The drawing under review shows one solid part. Ordinate dimensions are in mm from its lowest x, y, z. A direction names the side the tool comes from. Round coordinates to 2 decimals unless told otherwise and drop trailing zeros. Loops run counter-clockwise (first coordinate to the right, second up) from the corner with the lowest first, then second, coordinate; pieces in that order, holes last. Notation, with made-up numbers: M 9.5,-37 L 64.5,-37 A8 ccw 64.5,-23 Z; hole C 50.25,24.5 d11. An arc over 180 degrees is marked long. Use a Markdown table: item, result.
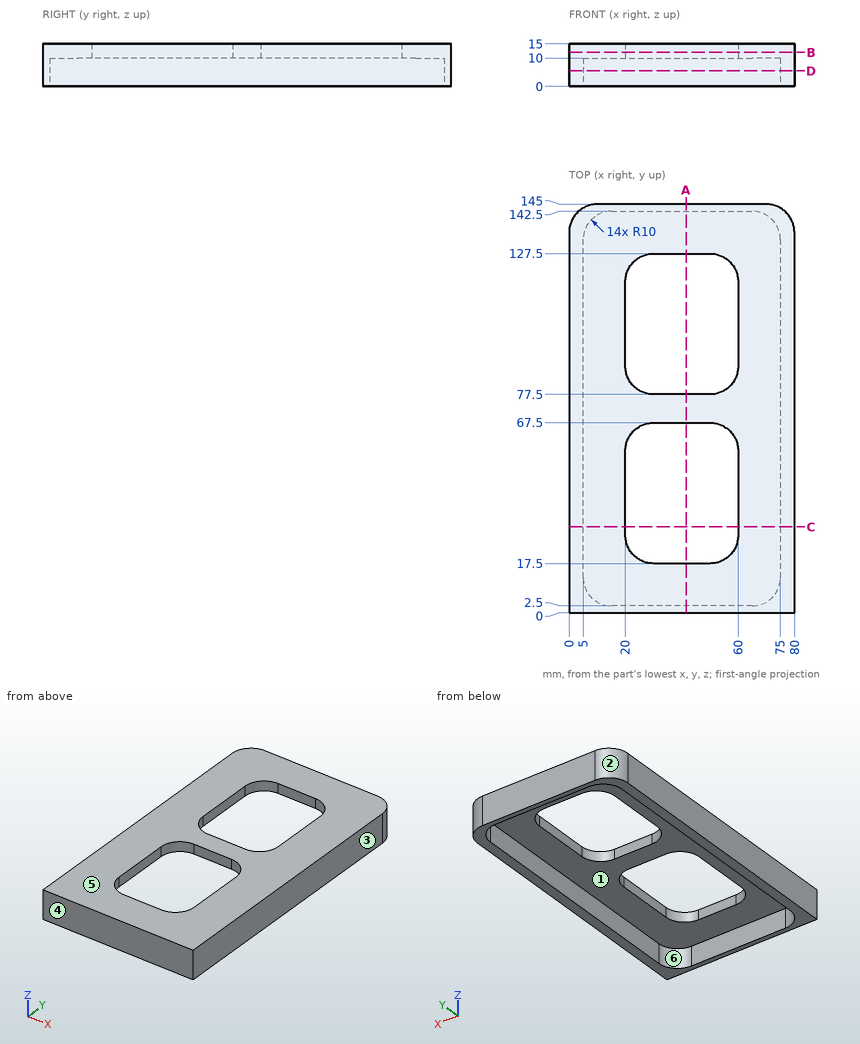
1. Machinability: for the marked faces 5 and 6, which of the approach directions +Z, -Z, +X, -X, +Y, -Y give a long, thin tool a straight path to every point of the face, cutting with its end or side? Answer none if there is none.
Check values:
| item | result |
|---|---|
| face 5 | +Z, +X, -X, +Y, -Y |
| face 6 | -Z |
2. The part is to be moulded in two halves that separate along X. For the marked faces 1, 2, 3 and 4, say which applies: pulls with the +X half, pulls with the -X half, needs draft (parallel to the pull), parting line crosses it, or undercut.
Check values:
| item | result |
|---|---|
| face 1 | undercut |
| face 2 | pulls with the -X half |
| face 3 | pulls with the +X half |
| face 4 | needs draft |
3. Take a section at A-A on x = 41.5. Give the boundary of the cut face in (y, z).
Check values:
| item | result |
|---|---|
| outline | M 0,0 L 2.5,0 L 2.5,10 L 17.5,10 L 17.5,15 L 0,15 Z; M 67.5,10 L 77.5,10 L 77.5,15 L 67.5,15 Z; M 127.5,10 L 142.5,10 L 142.5,0 L 145,0 L 145,15 L 127.5,15 Z |
4. Wall thickness on line 1 along Y through (x, z) = (41, 10.25); line 2 along X through (y, z) = (87.5, 1.5); line 3 along Y through (x, z) = (41, 6.25): over which ranges is each line inside the solid? List them lowest first. Write a range as from..to.
Check values:
| item | result |
|---|---|
| line 1 | y = 0..17.5, 67.5..77.5, 127.5..145 |
| line 2 | x = 0..5, 75..80 |
| line 3 | y = 0..2.5, 142.5..145 |
5. Insertion check: pin 1 (4 mm diameter, centred on x = 22.5, z = 5, fed in from -Y). The pin has a flat end and moves straight along its axis. Give the tip position at first contact, or say it passes through.
Check values:
| item | result |
|---|---|
| pin 1 | stops at y = 0 |
6. Take a section at D-D on z = 5.5. Give the boundary of the cut face in (x, y), and give its area (3 significant figures).
Check values:
| item | result |
|---|---|
| outline | M 0,0 L 80,0 L 80,135 A10 ccw 70,145 L 10,145 A10 ccw 0,135 Z; hole M 5,12.5 A10 ccw 15,2.5 L 65,2.5 A10 ccw 75,12.5 L 75,132.5 A10 ccw 65,142.5 L 15,142.5 A10 ccw 5,132.5 Z |
| area | 1,840 mm² |
7. Take a section at C-C on y = 30.5. Give the boundary of the cut face in (x, z), and give its area (3 significant figures).
Check values:
| item | result |
|---|---|
| outline | M 0,0 L 5,0 L 5,10 L 20,10 L 20,15 L 0,15 Z; M 60,10 L 75,10 L 75,0 L 80,0 L 80,15 L 60,15 Z |
| area | 300 mm² |
8. Take a section at B-B on z = 12. Give the boundary of the cut face in (x, y).
Check values:
| item | result |
|---|---|
| outline | M 0,0 L 80,0 L 80,135 A10 ccw 70,145 L 10,145 A10 ccw 0,135 Z; hole M 20,27.5 A10 ccw 30,17.5 L 50,17.5 A10 ccw 60,27.5 L 60,57.5 A10 ccw 50,67.5 L 30,67.5 A10 ccw 20,57.5 Z; hole M 20,87.5 A10 ccw 30,77.5 L 50,77.5 A10 ccw 60,87.5 L 60,117.5 A10 ccw 50,127.5 L 30,127.5 A10 ccw 20,117.5 Z |
